CAD build for the part. Positions are in the model's coordinates, mm. A direction names the side the tool comes from. Give positions to 0.01 mm unless a question says otherwise; leave off trailing zeros. Order: outer loops, then holes, each group sorted by start corner. A loop starts at its lowest first (then second) coordinate and runs counter-clockwise, first axis right, second up.
```python
from build123d import *

# Parameters (mm, degrees)
SKETCH_W        = 203
SKETCH_H        = 153
PAD_DEPTH       = 2
SKETCH002_W     = 20
SKETCH002_H     = 10
SKETCH002_W_2   = 22
SKETCH002_H_2   = 22
POCKET001_DEPTH = 2
SKETCH001_R     = 2.75
POCKET_DEPTH    = 2
SKETCH003_R     = 2
PAD001_DEPTH    = 2
SKETCH005_W     = 5
SKETCH005_H     = 5
PAD003_DEPTH    = 10
SKETCH006_W     = 2.5
SKETCH006_H     = 2.5
POCKET002_DEPTH = 5
SKETCH007_W     = 5
SKETCH007_H     = 5
PAD004_DEPTH    = 10
SKETCH008_W     = 2.5
SKETCH008_H     = 2.5
POCKET003_DEPTH = 5


with BuildPart() as part:
    # Sketch (on DatumPlane) → Pad (new body)
    with BuildSketch(Plane.XY.offset(-2)):
        Rectangle(SKETCH_W, SKETCH_H)
    extrude(amount=PAD_DEPTH)

    # Sketch002 (on DatumPlane) → Pocket001 (cut)
    with BuildSketch(Plane.XY):
        with Locations((0, -66.5)):
            Rectangle(SKETCH002_W, SKETCH002_H)
        with Locations((0, 64)):
            Rectangle(SKETCH002_W_2, SKETCH002_H_2)
    extrude(amount=-POCKET001_DEPTH, mode=Mode.SUBTRACT)

    # Sketch001 (on DatumPlane) → Pocket (cut)
    with BuildSketch(Plane.XY):
        with Locations((89, 64)):
            Circle(SKETCH001_R)
        with Locations((89, -64)):
            Circle(SKETCH001_R)
        with Locations((-89, -64)):
            Circle(SKETCH001_R)
        with Locations((-89, 64)):
            Circle(SKETCH001_R)
    extrude(amount=-POCKET_DEPTH, mode=Mode.SUBTRACT)

    # Sketch003 (on DatumPlane) → Pad001 (join)
    with BuildSketch(Plane.XY):
        with Locations((-16, 64)):
            Circle(SKETCH003_R)
        with Locations((16, 64)):
            Circle(SKETCH003_R)
    extrude(amount=PAD001_DEPTH)

    # Sketch005 (on DatumPlane) → Pad003 (join)
    with BuildSketch(Plane.XY):
        with Locations((-36.5, 14.5)):
            Rectangle(SKETCH005_W, SKETCH005_H)
        with Locations((12, 14.5)):
            Rectangle(SKETCH005_W, SKETCH005_H)
        with Locations((-36.5, -15)):
            Rectangle(SKETCH005_W, SKETCH005_H)
        with Locations((12, -15)):
            Rectangle(SKETCH005_W, SKETCH005_H)
    extrude(amount=PAD003_DEPTH)

    # Sketch006 (on Face39 of Pad003) → Pocket002 (cut)
    with BuildSketch(Plane.XY.offset(10)):
        with Locations((-35.25, 13.25)):
            Rectangle(SKETCH006_W, SKETCH006_H)
        with Locations((10.75, 13.25)):
            Rectangle(SKETCH006_W, SKETCH006_H)
        with Locations((10.75, -13.75)):
            Rectangle(SKETCH006_W, SKETCH006_H)
        with Locations((-35.25, -13.75)):
            Rectangle(SKETCH006_W, SKETCH006_H)
    extrude(amount=-POCKET002_DEPTH, mode=Mode.SUBTRACT)

    # Sketch007 (on DatumPlane) → Pad004 (join)
    with BuildSketch(Plane.XY):
        with Locations((24, -7)):
            Rectangle(SKETCH007_W, SKETCH007_H)
        with Locations((60, -7)):
            Rectangle(SKETCH007_W, SKETCH007_H)
        with Locations((24, -50)):
            Rectangle(SKETCH007_W, SKETCH007_H)
        with Locations((60, -50)):
            Rectangle(SKETCH007_W, SKETCH007_H)
    extrude(amount=PAD004_DEPTH)

    # Sketch008 (on Face63 of Pad004) → Pocket003 (cut)
    with BuildSketch(Plane.XY.offset(10)):
        with Locations((25.25, -8.25)):
            Rectangle(SKETCH008_W, SKETCH008_H)
        with Locations((58.75, -8.25)):
            Rectangle(SKETCH008_W, SKETCH008_H)
        with Locations((25.25, -48.75)):
            Rectangle(SKETCH008_W, SKETCH008_H)
        with Locations((58.75, -48.75)):
            Rectangle(SKETCH008_W, SKETCH008_H)
    extrude(amount=-POCKET003_DEPTH, mode=Mode.SUBTRACT)


solid = part.part
```
Item 1: Slice it at B-B (x = 89). Give the cut face in (y, z), and give its area (3 significant figures).
Item 2: Tool access for faces 1 (the face through (61, -47.5, 4)), 2 (the face through (14.5, 14, 5)), 3 (the face through (57.5, -51, 4)): list every direction of +Z, -Z, +X, -X, +Y, -Y with a clear straight run to the whole face (end or side of a thin tool).
Item 3: Slice it at D-D (z = 7.25). State how many separate pieces and enclosed holes the cut face has, and give its area (3 significant figures).
Item 4: Wall check: L1, parallel to Y at x = -89, z = -1.25; L2, parallel to X at y = -8.5, z = 5.5; L3, parallel to X at y = -50.5, z = 0.75. Give the ranges that are in metal, low to high.
Item 5: Two-plate mould, pull along X, no slides. Class faces 4 (the face through (16, 66, 1)), 5 (the face through (-39, 14, 5)), 6 (the face through (23, -47.5, 4)): released by +X, released by -X, zero draft, split by the parting line, or undercut.
Item 6: Slice it at A-A (y = -64). Give the cut face in (x, z).
Item 7: Drop flat-ended pins along their axis: pin 1 Ø6.5 at (x, y) = (-89, 64) entering from +Z; pin 2 Ø0.8 at (y, z) = (-14, 8) entering from -X; pin 3 Ø4 at (x, z) = (12, 5.5) entering from +Y. Give the stop position or say it passes through.
Item 8: Slice it at C-C (y = 57). Give the cut face in (x, z), and give its area (3 significant figures).
A:
1. outline: (-76.5, -2) - (-66.75, -2) - (-66.75, 0) - (-76.5, 0) - close; (-61.25, -2) - (61.25, -2) - (61.25, 0) - (-61.25, 0) - close; (66.75, -2) - (76.5, -2) - (76.5, 0) - (66.75, 0) - close
1. area: 284 mm2
2. face 1: +Z, +X, -X
2. face 2: +Z, +X, -Y
2. face 3: +Z, +Y, -Y
3. separate pieces: 8
3. enclosed holes: 0
3. area: 150 mm2
4. L1: y = -76.5 to -66.75, -61.25 to 61.25, 66.75 to 76.5
4. L2: x = 21.5 to 24, 60 to 62.5
4. L3: x = 21.5 to 26.5, 57.5 to 62.5
5. face 4: undercut
5. face 5: released by -X
5. face 6: zero draft
6. outline: (-101.5, -2) - (-91.75, -2) - (-91.75, 0) - (-101.5, 0) - close; (-86.25, -2) - (-10, -2) - (-10, 0) - (-86.25, 0) - close; (10, -2) - (86.25, -2) - (86.25, 0) - (10, 0) - close; (91.75, -2) - (101.5, -2) - (101.5, 0) - (91.75, 0) - close
7. pin 1: stops at z = 0
7. pin 2: stops at x = -39
7. pin 3: stops at y = 17
8. outline: (-101.5, -2) - (-11, -2) - (-11, 0) - (-101.5, 0) - close; (11, -2) - (101.5, -2) - (101.5, 0) - (11, 0) - close
8. area: 362 mm2
